Input: part model. Units: mm. Frame: model coordinates. A direction names the side the tool comes from. Coordinates: 2 decimals unless noted, no trailing zeros. Write each loop counter-clockwise with the first axis right and the second up, starting at its lowest first coordinate (ties: lowest second). Pieces come first, ordered by that corner, then holes. Notation, with made-up numbers: M 66,77 L 104,77 A12 cw 104,97 Z; hole C 23.25,29.25 d11. An arc over 180 degrees is marked long. Use CSV: the item, a comma, the result in double quotes.
```python
from build123d import *

# Parameters (mm, degrees)
SKETCH_1_W          = 115
SKETCH_1_H          = 54
SKETCH_1_R          = 2
SKETCH_1_W_2        = 40
SKETCH_1_H_2        = 20
EXTRUDE_3_DEPTH     = 5
SKETCH_3_R          = 1.75
CUT_EXTRUDE_2_DEPTH = 15
CUT_EXTRUDE_3_DEPTH = 10
SKETCH_5_R          = 1.7
CUT_EXTRUDE_4_DEPTH = 10


with BuildPart() as part:
    # 草圖1 → 填料-伸長3 (new body)
    with BuildSketch(Plane.XY):
        with Locations((13.062480584, -3.484099434)):
            Rectangle(SKETCH_1_W, SKETCH_1_H)
        with Locations((-0.937519416, -8.484099434)):
            Circle(SKETCH_1_R, mode=Mode.SUBTRACT)
        with Locations((47.062480584, -8.484099434)):
            Circle(SKETCH_1_R, mode=Mode.SUBTRACT)
        with Locations((-0.937519416, 1.515900566)):
            Circle(SKETCH_1_R, mode=Mode.SUBTRACT)
        with Locations((47.062480584, 1.515900566)):
            Circle(SKETCH_1_R, mode=Mode.SUBTRACT)
        with Locations((23.062480584, -3.484099434)):
            Rectangle(SKETCH_1_W_2, SKETCH_1_H_2, mode=Mode.SUBTRACT)
    extrude(amount=EXTRUDE_3_DEPTH)

    # 草圖3 → 除料-伸長2 (cut)
    with BuildSketch(Plane.XZ.offset(30.484099434)):
        with Locations(Location((29.062480584, 2.5, 0), (0, 0, 270))):
            Circle(SKETCH_3_R)
        with Locations(Location((-2.937519416, 2.5, 0), (0, 0, 270))):
            Circle(SKETCH_3_R)
    extrude(amount=-CUT_EXTRUDE_2_DEPTH, mode=Mode.SUBTRACT)

    # 草圖4 → 除料-伸長3 (cut)
    with BuildSketch(Plane.XY.offset(5)):
        Polygon((0.340707034, -3.484099434), (3.062480584, -6.205872984), (3.062480584, -0.762325884), align=None)
    extrude(amount=-CUT_EXTRUDE_3_DEPTH, mode=Mode.SUBTRACT)

    # 草圖5 → 除料-伸長4 (cut)
    with BuildSketch(Plane(origin=(0, 23.515900566, 0), x_dir=(1, 0, 0), z_dir=(0, 1, 0))):
        with Locations(Location((60.562480584, -2.5, 0), (0, 0, 270))):
            Circle(SKETCH_5_R)
        with Locations(Location((-34.437519416, -2.5, 0), (0, 0, 270))):
            Circle(SKETCH_5_R)
    extrude(amount=-CUT_EXTRUDE_4_DEPTH, mode=Mode.SUBTRACT)


solid = part.part
```
1. Mould query, pull axis Z, two halves, no side actions, for faces 1 (the flat face through (-3, -15.484, 3)), 2 (the cylindrical face through (58.903, 18.586, 2.131)), 3 (the flat face through (-1, -3, 5)), 4 (the cylindrical face through (48.97, -7.88, 2.46)). Classes: pulls with the +Z half, pulls with the -Z half, needs draft (parallel to the pull), parting line crosses it, or undercut.
Resolved:
face 1,"undercut"
face 2,"undercut"
face 3,"pulls with the +Z half"
face 4,"needs draft"
2. Contact query for flat-ended pins moving along their axis: pin 1 Ø3 at (x, y) = (-0.94, 1.52) entering from +Z; pin 2 Ø2 at (x, z) = (60.56, 2.5) entering from +Y; pin 3 Ø1.8 at (x, z) = (-3, 2) entering from -Y. Output: stop coordinate, or through.
Resolved:
pin 1,"passes through"
pin 2,"stops at y = 13.52"
pin 3,"stops at y = -15.48"
3. Section B-B (z = 3.1). State how many separate pieces and enclosed holes the cut face has, then the cut area to 3 significant figures.
Resolved:
separate pieces,"1"
enclosed holes,"5"
area,"5,190 mm^2"
4. Material intervals for line 1 (X direction, y = 21, z = 2.5); line 2 (Y direction, x = 36, z = 3.65); line 3 (X direction, y = 5, z = 2.9), sorted ascending. Write a range as [from, to].
Resolved:
line 1,"x = [-44.44, -36.14], [-32.74, 58.86], [62.26, 70.56]"
line 2,"y = [-30.48, -13.48], [6.52, 23.52]"
line 3,"x = [-44.44, 3.06], [43.06, 70.56]"
5. Section A-A (x = 37). Return loops of the section in (y, z).
Resolved:
outline,"M -30.48,0 L -13.48,0 L -13.48,5 L -30.48,5 Z; M 6.52,0 L 23.52,0 L 23.52,5 L 6.52,5 Z"
6. Access query for faces 5 (the flat face through (43.062, -4, 2)), 6 (the flat face through (-34, 13.516, 2)), 7 (the cylindrical face through (30.8, -23.1, 2.7)), 8 (the flat face through (12, 23.516, 2)), 9 (the flat face through (-44.438, -4, 2)). Directions: +Z, -Z, +X, -X, +Y, -Y. A direction counts if a zero-diameter tool reaches every point of the face in a straight line with its end or side. Return the directions, or none.
Resolved:
face 5,"+Z, -Z"
face 6,"+Y"
face 7,"-Y"
face 8,"+Z, -Z, +X, -X, +Y"
face 9,"+Z, -Z, -X, +Y, -Y"
7. Section C-C (y = 15.5). Return loops of the section in (x, z).
Resolved:
outline,"M -44.44,0 L 70.56,0 L 70.56,5 L -44.44,5 Z; hole C -34.44,2.5 d3.4; hole C 60.56,2.5 d3.4"
